Can you work these out from the model? Positions are in its coordinate system, mm. A direction names the side the tool comes from. Give positions to 0.01 mm unless a question says otherwise; leave off trailing zeros. Loops run counter-clockwise (first coordinate to the right, second up) from the corner with the lowest first, then second, coordinate; pieces in that order, holes last. Notation, with made-up numbers: (43.5, 32) - (94.5, 32) arc R12 cw to (94.5, 49) - close; hole circle Ø11 at (-13, 48.25). An arc over 180 degrees is marked (long way). Answer as a JSON object with one key per item and string values. Group by question number.
Item 1: Which directions (+Z, -Z, +X, -X, +Y, -Y) give clear straight access to the entire face, cutting with the end or side of a thin tool? Please do faces 1 (the flat face through (2, 0, 1)), 2 (the flat face through (3, 25, 1)), 3 (the flat face through (1, 50, 1)), 4 (the flat face through (29, 56, 1)), 5 (the flat face through (29, 25, 1)).
Item 2: Will these pins go through, and if not, where does the flat tip stop? pin 1 (0.9 mm diameter, centred on y = -5.5, z = 1, fed in from +X); pin 2 (0.9 mm diameter, centred on y = 55.5, z = 1.5, fed in from -X); pin 3 (1.5 mm diameter, centred on x = 1, z = 2, fed in from +Y).
Item 3: Suppose I cut it at D-D on y = 14. Write out the boundary of the cut face in (x, z).
Item 4: Please list where these lines run through material, in increasing order: L1, parallel to Y at x = 11.5, z = 0.3; L2, parallel to X at y = 17.5, z = 0.8.
Item 5: Suppose I cut it at B-B on z = 0.7. Write out the boundary of the cut face in (x, y), and give its area (3 significant figures).
Item 6: Thinking about a two-plate mould opening in X: for faces 6 (the flat face through (23, 26, 3)), 7 (the flat face through (10.5, 25, 1)), 8 (the flat face through (3, -5, 1)), 9 (the flat face through (16, 26.5, 1)), which applies, pulls with the +X half, pulls with the -X half, needs draft (parallel to the pull), parting line crosses it, or undercut?
Item 7: Suppose I cut it at A-A on y = 25. Write out the boundary of the cut face in (x, z), and give its area (3 significant figures).
Item 8: Suppose I cut it at C-C on x = 19. Write out the boundary of the cut face in (y, z).
Autodesk Inventor part; units mm, degrees
ref_plane "YZ Plane" through (0, 0, 0) normal (1, 0, 0) x (0, 1, 0)
ref_plane "XZ Plane" through (0, 0, 0) normal (0, 1, 0) x (-1, 0, 0)
ref_plane "XY Plane" through (0, 0, 0) normal (0, 0, 1) x (1, 0, 0)
sketch "Sketch1" plane through (0, 0, 0) normal (0, 0, 1) x (1, 0, 0)
  line L0 (0, 0) -> (0, 10)
  line L1 (0, 10) -> (3, 10)
  line L2 (3, 10) -> (3, 40)
  line L3 (3, 40) -> (0, 40)
  line L4 (0, 40) -> (0, 50)
  line L5 (32, 50) -> (32, 40)
  line L6 (32, 40) -> (29, 40)
  line L7 (29, 40) -> (29, 10)
  line L8 (29, 10) -> (32, 10)
  line L9 (32, 10) -> (32, 0)
  line L10 (10.5, 23.5) -> (20.5, 23.5)
  line L11 (20.5, 23.5) -> (20.5, 26.5)
  line L12 (20.5, 26.5) -> (10.5, 26.5)
  line L13 (10.5, 26.5) -> (10.5, 23.5)
  line L14 (3, 50) -> (3, 61)
  line L15 (3, 61) -> (29, 61)
  line L16 (29, 61) -> (29, 50)
  line L17 (3, 0) -> (3, -11)
  line L18 (3, -11) -> (29, -11)
  line L19 (29, -11) -> (29, 0)
  line L20 (0, 50) -> (3, 50)
  line L21 (29, 50) -> (32, 50)
  line L22 (32, 0) -> (29, 0)
  line L23 (3, 0) -> (0, 0)
  dimension "d19" = 10
  dimension "d20" = 3
  dimension "d22" = 10
  dimension "d23" = 3
  dimension "d24" = 30
  dimension "d25" = 3
  dimension "d26" = 10
  dimension "d27" = 32
  dimension "d28" = 10
  dimension "d29" = 3
  dimension "d30" = 3
  dimension "d31" = 10
  dimension "d32" = 7.5
  dimension "d35" = 30
  dimension "d36" = 72
  dimension "d39" = 34.5
  dimension "d40" = 26
  dimension "d41" = 26
  dimension "d42" = 11
  dimension "d43" = 11
extrude "Extrusion1" add sketch "Sketch1" along normal blind 3
properties part number "OpenROV 2.3 Dev EChassis Light Plate"
Worked out:
{
 "1": {"face 1": "+Z, -Z, -X, -Y", "face 2": "+Z, -Z, -X", "face 3": "+Z, -Z, -X, +Y", "face 4": "+Z, -Z, +X, +Y", "face 5": "+Z, -Z, +X"},
 "2": {"pin 1": "stops at x = 29", "pin 2": "stops at x = 3", "pin 3": "stops at y = 50"},
 "3": {"outline": "(3, 0) - (29, 0) - (29, 3) - (3, 3) - close"},
 "4": {"L1": "y = -11 to 23.5, 26.5 to 61", "L2": "x = 3 to 29"},
 "5": {"outline": "(0, 0) - (3, 0) - (3, -11) - (29, -11) - (29, 0) - (32, 0) - (32, 10) - (29, 10) - (29, 40) - (32, 40) - (32, 50) - (29, 50) - (29, 61) - (3, 61) - (3, 50) - (0, 50) - (0, 40) - (3, 40) - (3, 10) - (0, 10) - close; hole (10.5, 23.5) - (20.5, 23.5) - (20.5, 26.5) - (10.5, 26.5) - close", "area": "1,960 mm2"},
 "6": {"face 6": "needs draft", "face 7": "undercut", "face 8": "pulls with the -X half", "face 9": "undercut"},
 "7": {"outline": "(3, 0) - (10.5, 0) - (10.5, 3) - (3, 3) - close; (20.5, 0) - (29, 0) - (29, 3) - (20.5, 3) - close", "area": "48.0 mm2"},
 "8": {"outline": "(-11, 0) - (23.5, 0) - (23.5, 3) - (-11, 3) - close; (26.5, 0) - (61, 0) - (61, 3) - (26.5, 3) - close"}
}
